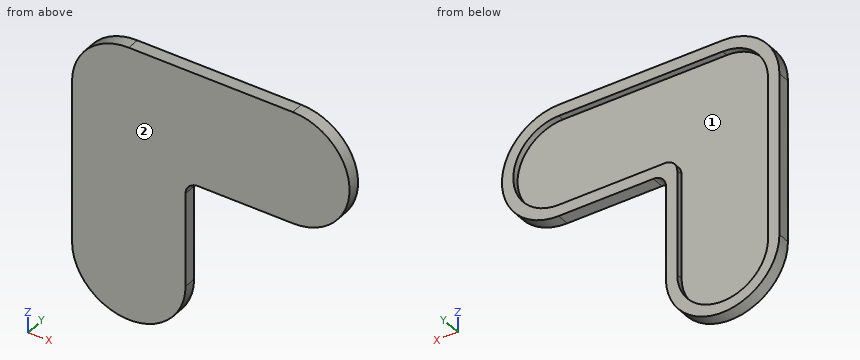
```python
from build123d import *

# Parameters (mm, degrees)
BOSS_EXTRUDE1_DEPTH = 10
CUT_EXTRUDE1_START  = -5
CUT_EXTRUDE1_DEPTH  = 5
FILLET1_R           = 10
FILLET2_R           = 10


# Read off the part's stored shape, not the designer's step: Cut-Extrude1
with BuildPart() as part:
    # Sketch1 → Boss-Extrude1 (new body)
    with BuildSketch(Plane(origin=(0, 0, 0), x_dir=(1, 0, 0), z_dir=(0, 1, 0))):
        with BuildLine():
            ThreePointArc((130, -45.182255659), (175, -0.182255659), (130, 44.817744341))
            Line((130, 44.817744341), (44.916086644, 44.937029146))
            Line((44.916086644, 44.937029146), (45, 130))
            ThreePointArc((45, 130), (0, 175), (-45, 130))
            Line((-45, 130), (-45, 0))
            ThreePointArc((-45, 0), (-31.819805153, -31.819805153), (0, -45))
            Line((0, -45), (130, -45.182255659))
        make_face()
    extrude(amount=BOSS_EXTRUDE1_DEPTH)

    # Cut-Extrude1 outline → Cut-Extrude1 (cut)
    with BuildSketch(Plane(origin=(0, 10, 0), x_dir=(1, 0, 0), z_dir=(0, 1, 0)).offset(CUT_EXTRUDE1_START)):
        with BuildLine():
            Line((36, 35.949529202), (36, 130))
            ThreePointArc((36, 130), (0, 166), (-36, 130))
            Line((-36, 130), (-36, 0))
            ThreePointArc((-36, 0), (-25.455844123, -25.455844123), (0, -36))
            Line((0, -36), (130, -36.182255659))
            ThreePointArc((130, -36.182255659), (166, -0.182255659), (130, 35.817744341))
            Line((130, 35.817744341), (36, 35.949529202))
        make_face()
    extrude(amount=CUT_EXTRUDE1_DEPTH, mode=Mode.SUBTRACT)

    # Fillet1
    fillet1_edges = [part.edges().sort_by_distance(p)[0] for p in [
        (44.916086644, 5, -44.937029146),
    ]]
    fillet(fillet1_edges, radius=FILLET1_R)

    # Fillet2
    fillet2_edges = [part.edges().sort_by_distance(p)[0] for p in [
        (36, 7.5, -35.949529202),
    ]]
    fillet(fillet2_edges, radius=FILLET2_R)


solid = part.part
```
Verification items for the finished model (mm, model axes). Face numbers are marked on the shaded views. Coordinates: 2 decimals unless noted, no trailing zeros. Write each loop counter-clockwise with the first axis right and the second up, starting at its lowest first coordinate (ties: lowest second). Pieces come first, ordered by that corner, then holes. Notation, with made-up numbers: M 34.25,69.5 L 45.25,69.5 A23 cw 45.25,103.5 Z; hole C 65,53.25 d3. An arc over 180 degrees is marked long. Answer as a JSON object with one key per item and string values. Group by question number.
(1) Cross-section at B-B, the plane z = -140. Record the cut outline in (x, y).
(2) Material ranges on line 1 (Z direction, x = 117, y = 8); line 2 (Z direction, x = 104, y = 5.5); line 3 (Z direction, x = 98, y = 1.5), recorded low to high.
(3) Release check for a two-part mould opening along Z. For the marked faces 1 and 2 record: +Z half, -Z half, draft (parallel to the pull), parting line (faces both ways), or undercut.
(4) Gauge pin test, flat ends, axial feed: pin 1 (4 mm diameter, centred on y = 6.5, z = -92, fed in from +X); pin 2 (4 mm diameter, centred on x = 54.5, y = 1.5, fed in from -Z); pin 3 (1.5 mm diameter, centred on y = 5.5, z = -70, fed in from +X); pin 4 (8 mm diameter, centred on x = -6.5, z = -110, fed in from -Y). Record the tip position at first contact, or that the pin passes through.
(5) Cross-section at A-A, the plane y = 3.5. Record the cut outline in (x, z), and give its area (3 significant figures).
Reply:
{
 "1": {"outline": "M -43.87,0 L 43.87,0 L 43.87,10 L 34.58,10 L 34.58,5 L -34.58,5 L -34.58,10 L -43.87,10 Z"},
 "2": {"line 1": "-44.84 to -35.84, 36.16 to 45.16", "line 2": "-44.85 to -35.85, 36.15 to 45.15", "line 3": "-44.86 to 45.14"},
 "3": {"face 1": "undercut", "face 2": "draft"},
 "4": {"pin 1": "x = 44.96", "pin 2": "z = -45.22", "pin 3": "x = 44.94", "pin 4": "y = 0"},
 "5": {"outline": "M -45,-130 A45 ccw 45,-130 L 44.93,-54.93 A10 cw 54.91,-44.92 L 130,-44.82 A45 ccw 130,45.18 L 0,45 A45 ccw -45,0 Z", "area": "29,300 mm²"}
}
